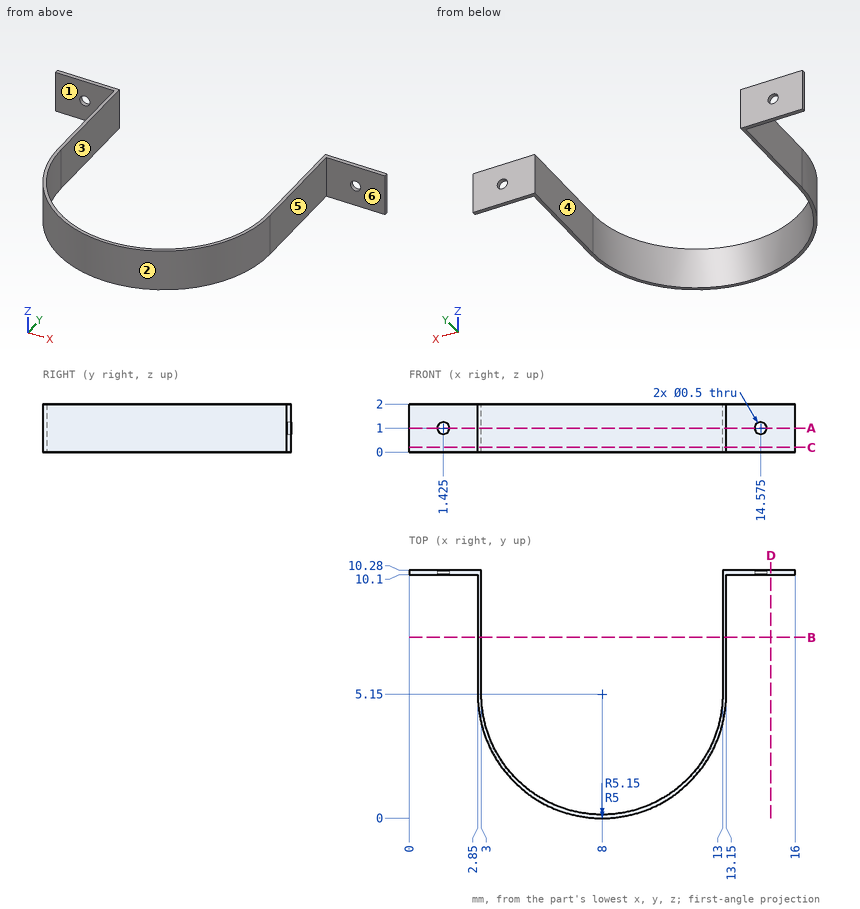
Print and shaded views of the part. All mm, measured from the part's lowest x, y and z. A direction names the side the tool comes from. Round coordinates to 2 decimals unless told otherwise and drop trailing zeros. Write each loop counter-clockwise with the first axis right and the second up, starting at its lowest first coordinate (ties: lowest second). Pieces come first, ordered by that corner, then holes. Notation, with made-up numbers: (62, -9) -> (118, -9) arc R8 cw to (118, -1) -> close; hole circle Ø10 at (2.25, -4). An arc over 180 degrees is marked (long way). Return JSON: item names as keys, results as strings. Group by question number.
Q1. Mould opens along X. For the marked faces 4, 5 and 6 say: pulls with the +X half, pulls with the -X half, needs draft (parallel to the pull), parting line crosses it, or undercut.
Q2. Saw through at C-C on z = 0.2. Write the cut outline in (x, y), plus the area to 3 significant figures.
Q3. Saw through at B-B on y = 7.5. Write the cut outline in (x, z).
Q4. Pin check, flat tips, straight feed: pin 1 (1 mm diameter, centred on x = 5, z = 1, fed in from +Y); pin 2 (1 mm diameter, centred on x = 1, z = 1.5, fed in from -Y); pin 3 (1 mm diameter, centred on y = 7.5, z = 1, fed in from -X); pin 4 (3 mm diameter, centred on x = 5.5, y = 6.5, fed in from +Z). Stop position of each tip, or through.
Q5. Probe L1, parallel to X at y = 10.2, z = 1 (3 decimals); L2, parallel to Y at x = 1, z = 0.2; L3, parallel to X at y = 1.25, z = 0.75. List the from-to ranges inside material, lowest first. Write a range as [from, to].
Q6. Saw through at D-D on x = 15. Write the cut outline in (y, z).
Q7. Saw through at A-A on z = 1. Write the cut outline in (x, y) (3 decimals), plus the area to 3 significant figures.
Q8. Which spindle directions (+Z, -Z, +X, -X, +Y, -Y) get a long thin tool onto all of the face, cutting with end or side? Do the marked faces 1, 2 and 3. Say none if no direction does.
Answer:
{
 "1": {"face 4": "undercut", "face 5": "pulls with the +X half", "face 6": "needs draft"},
 "2": {"outline": "(0, 10.1) -> (2.85, 10.1) -> (2.85, 5.15) arc R5.15 ccw to (13.15, 5.15) -> (13.15, 10.1) -> (16, 10.1) -> (16, 10.28) -> (13, 10.28) -> (13, 5.15) arc R5 cw to (3, 5.15) -> (3, 10.28) -> (0, 10.28) -> close", "area": "4.96 mm2"},
 "3": {"outline": "(2.85, 0) -> (3, 0) -> (3, 2) -> (2.85, 2) -> close; (13, 0) -> (13.15, 0) -> (13.15, 2) -> (13, 2) -> close"},
 "4": {"pin 1": "y = 1.58", "pin 2": "y = 10.1", "pin 3": "x = 2.85", "pin 4": "through"},
 "5": {"L1": "[0, 1.175], [1.675, 3], [13, 14.325], [14.825, 16]", "L2": "[10.1, 10.28]", "L3": "[4.64, 4.87], [11.13, 11.36]"},
 "6": {"outline": "(10.1, 0) -> (10.28, 0) -> (10.28, 2) -> (10.1, 2) -> close"},
 "7": {"outline": "(0, 10.1) -> (1.175, 10.1) -> (1.175, 10.28) -> (0, 10.28) -> close; (1.675, 10.1) -> (2.85, 10.1) -> (2.85, 5.15) arc R5.15 ccw to (13.15, 5.15) -> (13.15, 10.1) -> (14.325, 10.1) -> (14.325, 10.28) -> (13, 10.28) -> (13, 5.15) arc R5 cw to (3, 5.15) -> (3, 10.28) -> (1.675, 10.28) -> close; (14.825, 10.1) -> (16, 10.1) -> (16, 10.28) -> (14.825, 10.28) -> close", "area": "4.78 mm2"},
 "8": {"face 1": "+Z, -Z, -X, -Y", "face 2": "+Z, -Z, -Y", "face 3": "+Z, -Z, +Y"}
}
